from build123d import *

# Parameters (mm, degrees)
F0_W     = 304.8
F0_H     = 12.7
F0_W_2   = 25.4
F0_H_2   = 76.2
F2_DEPTH = 12.7
F3_SIZE2 = 94.794081
F3_SIZE  = 25.39999
F4_R     = 20.3093495569
F4_W     = 25.4
F4_H     = 25.4
F5_DEPTH = 18.288
F6_R     = 9.4776416284
F7_DEPTH = 25.4


# Not quite as in the source:
# - a fillet or chamfer is up to 0.001 mm smaller than in the source, because OpenCascade refuses the exact size


with BuildPart() as f1:
    # F0 (on Front) → F1 (revolve)
    with BuildSketch(Plane.XZ):
        with Locations((121.4729587615, 6.35)):
            Rectangle(F0_W, F0_H)
    revolve(axis=Axis((121.4729587615, 0, 0), (1, 0, 0)))

    # F0 (on Front) → F2 (join, symmetric)
    with BuildSketch(Plane.XZ):
        Polygon((-56.3270412385, 0), (-30.9270412385, 0), (-30.9270412385, 12.7), (-30.9270412385, 50.8), (-56.3270412385, 50.8), align=None)
        with Locations((-43.6270412385, -38.1)):
            Rectangle(F0_W_2, F0_H_2)
    extrude(amount=F2_DEPTH, both=True)

    # F3 (size 25.4 and 94.7940905122 in the source; OpenCascade refuses exactly that, so slightly less here)
    f3_edges = [f1.edges().sort_by_distance(p)[0] for p in [
        (-56.327041, 0, -76.2),
    ]]
    f3_side = f1.faces().sort_by_distance((-43.627041, 0, -76.2))[0]
    chamfer(f3_edges, length=F3_SIZE, length2=F3_SIZE2, reference=f3_side)

    # F4 (on face) → F5 (join)
    with BuildSketch(Plane.XY.offset(50.8)):
        with Locations((-43.6270412385, 0)):
            Circle(F4_R)
        with Locations((-43.6270412385, 0)):
            Rectangle(F4_W, F4_H, mode=Mode.SUBTRACT)
        with Locations((-43.6270412385, 0)):
            Rectangle(F4_W, F4_H)
    extrude(amount=F5_DEPTH)

    # F6 (on face) → F7 (cut)
    with BuildSketch(Plane.XZ.offset(12.7)):
        with Locations((-43.4236600995, 27.4490546435)):
            Circle(F6_R)
    extrude(amount=-F7_DEPTH, mode=Mode.SUBTRACT)


solid = f1.part
Here's how the part is built. I have some questions about the finished solid (model axes, mm). A direction names the side the tool comes from. Give positions to 0.01 mm unless a question says otherwise; leave off trailing zeros. Write each loop counter-clockwise with the first axis right and the second up, starting at its lowest first coordinate (ties: lowest second). Pieces come first, ordered by that corner, then holes. Notation, with made-up numbers: (5.25, 12.25) -> (13.25, 12.25) arc R24 ccw to (13.25, 47.25) -> close; hole circle Ø1 at (26, -33.75). An arc over 180 degrees is marked (long way). Use one line per item in the form item = value. Start each with the question number.
1. Imagine slicing it at B-B on x = 183. List the corners of the cut face in (y, z) for me, plus the area to 3 significant figures.
2. Thinking about a two-plate mould opening in Z: for faces 5 (the face through (-30.927, 0, -39)), 6 (the face through (-44, 0, 69.088)), 7 (the face through (-43.805, 0.178, -28.139)), 8 (the face through (-38.33, -0.18, 35.44)), which applies, +Z half, -Z half, draft (parallel to the pull), parting line (faces both ways), or undercut?
3. Imagine slicing it at D-D on z = 6. List the corners of the cut face in (x, y) for me, plus the area to 3 significant figures.
4. On a 3-axis mill with a long thin cutter (end or side, diameter ignored), from which of +Z, -Z, +X, -X, +Y, -Y can I reach the whole of each face in a straight line? I mean faces 1 (the face through (-58.596, 13.726, 59.816)), 2 (the face through (123.61, 12.4, -2.75)), 3 (the face through (-41, -12.7, 2)), 4 (the face through (-41, 12.7, 2)). Say none if no direction works.
5. If I drill on L1, parallel to Y at x = -34.5, z = 6; L2, parallel to Z at x = 255.5, y = 1; L3, parallel to Z at x = 116, y = 3.5, over which ranges is the centre line in solid material (lowest first)?
6. Imagine slicing it at C-C on z = 44.5. List the corners of the cut face in (x, y) for me.
7. Will these pins go through, and if not, where does the flat tip stop? pin 1 Ø6 at (x, y) = (204, 7) entering from -Z; pin 2 Ø7.5 at (x, z) = (-43, 17.5) entering from +Y; pin 3 Ø10 at (y, z) = (1, 44) entering from -X.
Entries:
q1.outline = circle Ø25.4 at (0, 0)
q1.area = 507 mm²
q2.face_5 = draft
q2.face_6 = +Z half
q2.face_7 = -Z half
q2.face_8 = undercut
q3.outline = (-52.95, -12.7) -> (-30.93, -12.7) -> (-30.93, -11.19) -> (273.87, -11.19) -> (273.87, 11.19) -> (-30.93, 11.19) -> (-30.93, 12.7) -> (-52.95, 12.7) -> close
q3.area = 7,380 mm²
q4.face_1 = +Z
q4.face_2 = +X
q4.face_3 = -Z, +X, -X, -Y
q4.face_4 = -Z, +X, -X, +Y
q5.L1 = -12.7 to 12.7
q5.L2 = -12.66 to 12.66
q5.L3 = -12.21 to 12.21
q6.outline = (-56.33, -12.7) -> (-30.93, -12.7) -> (-30.93, 12.7) -> (-56.33, 12.7) -> close
q7.pin_1 = -12.05
q7.pin_2 = 12.7
q7.pin_3 = -56.33
